For this review, take the finished solid that the model builds, in its own axes (mm). Face numbers are marked on the shaded views. Give positions to 0.01 mm unless a question says otherwise; leave off trailing zeros. Order: outer loops, then holes, each group sorted by start corner. A loop starts at its lowest first (then second) coordinate and runs counter-clockwise, first axis right, second up.
Autodesk Inventor part; units mm, degrees
ref_plane "Work Plane1" through (15.24, 0, -4.7625) normal (0, 0, 1) x (1, 0, 0)
ref_plane "YZ Plane" through (0, 0, 0) normal (1, 0, 0) x (0, 1, 0)
ref_plane "XZ Plane" through (0, 0, 0) normal (0, 1, 0) x (-1, 0, 0)
sketch "Sketch1" plane through (0, 0, 0) normal (0, 1, 0) x (-1, 0, 0)
  line L0 (0, 0) -> (0, -9.525)
  line L1 (-15.24, 4.2545) -> (-15.24, -13.7795)
  line L2 (0, 0) -> (-15.24, 4.2545)
  line L3 (0, -9.525) -> (-15.24, -13.7795)
  line L4 (-15.24, 4.2545) -> (-19.05, 4.2545)
  line L5 (-19.05, 4.2545) -> (-19.05, 2.9845)
  line L6 (-19.05, 2.9845) -> (-15.24, 2.9845)
  line L7 (-15.24, 2.9845) -> (-15.24, 4.2545)
  line L8 (-15.24, -13.7795) -> (-19.05, -13.7795)
  line L9 (-19.05, -13.7795) -> (-19.05, -12.5095)
  line L10 (-19.05, -12.5095) -> (-15.24, -12.5095)
  line L11 (-15.24, -12.5095) -> (-15.24, -13.7795)
  line L12 (0, 0) -> (0, 3.175)
  line L13 (-15.24, 4.2545) -> (-15.24, 7.4295)
  line L14 (0, -9.525) -> (0, -12.7)
  line L15 (-15.24, -13.7795) -> (-15.24, -16.9545)
  line L16 (-15.24, -16.9545) -> (0, -12.7)
  line L17 (0, 3.175) -> (-15.24, 7.4295)
  line L18 (-15.24, 7.4295) -> (-34.29, 7.4295)
  line L19 (-19.05, 4.2545) -> (-34.29, 4.2545)
  line L20 (-34.29, 4.2545) -> (-34.29, 7.4295)
  line L21 (-15.24, -16.9545) -> (-34.29, -16.9545)
  line L22 (-34.29, -16.9545) -> (-34.29, -13.7795)
  line L23 (-34.29, -13.7795) -> (-19.05, -13.7795)
  line L24 (-34.29, 7.4295) -> (-37.465, 7.4295)
  line L25 (-37.465, 7.4295) -> (-37.465, -17.5895)
  line L26 (-37.465, -17.5895) -> (-34.29, -17.5895)
  line L27 (-34.29, -17.5895) -> (-34.29, 7.4295)
  line L28 (-15.24, -13.7795) -> (-34.29, -13.7795)
  line L29 (-34.29, -13.7795) -> (-34.29, 4.2545)
  line L30 (-34.29, 4.2545) -> (-15.24, 4.2545)
  line L31 (-15.24, 4.2545) -> (-15.24, -13.7795)
  line L32 (-15.24, 4.2545) -> (-34.29, 4.2545)
  line L33 (-34.29, 4.2545) -> (-34.29, 7.4295)
  line L34 (-34.29, 7.4295) -> (-15.24, 7.4295)
  line L35 (-15.24, 7.4295) -> (-15.24, 4.2545)
  line L36 (-15.24, -7.5565) -> (-22.86, -7.5565)
  line L37 (-22.86, -7.5565) -> (-22.86, -1.9685)
  line L38 (-22.86, -1.9685) -> (-15.24, -1.9685)
  line L39 (-15.24, -1.9685) -> (-15.24, -7.5565)
  dimension "d0" = 9.525
  dimension "d1" = 15.24
  dimension "d2" = 18.034
  dimension "d3" = 4.2545
  dimension "d4" = 3.81
  dimension "d5" = 1.27
  dimension "d6" = 3.81
  dimension "d7" = 1.27
  dimension "d8" = 3.175
  dimension "d9" = 3.175
  dimension "d10" = 3.175
  dimension "d11" = 3.175
  dimension "d12" = 19.05
  dimension "d13" = 3.175
  dimension "d30" = 7.62
  dimension "d31" = 5.588
  dimension "d32" = 6.223
extrude "Extrusion6" add sketch "Sketch1" along normal blind 5.588 contours L0 L3 L1 L2 | L1 L36 L37 L38
sketch "Sketch5" plane through (0, 5.588, 0) normal (0, 1, 0) x (1, 0, 0)
  circle A0 centre (8.636, 4.7625) radius 1.5875
  line L0 (0, 9.525) -> (0, 0)
  dimension "d35" = 3.175
  dimension "d36" = 8.636
extrude "Extrusion7" cut sketch "Sketch5" against normal blind 5.588
sketch "Sketch6" plane through (15.24, 0, 4.2545) normal (1, 0, 0) x (0, 0, -1)
  line L0 (6.223, 0) -> (6.223, 5.588)
  line L1 (0, 5.588) -> (6.223, 5.588)
  line L2 (0, 0) -> (0, 5.588)
  line L3 (0, 0) -> (6.223, 0)
  line L4 (11.811, 5.588) -> (11.811, 0)
  line L5 (11.811, 0) -> (18.034, 0)
  line L6 (18.034, 0) -> (18.034, 5.588)
  line L7 (11.811, 5.588) -> (18.034, 5.588)
  circle A0 centre (1.863, 2.794) radius 0.381
  circle A1 centre (4.4524, 2.794) radius 0.381
  line L8 (6.223, 5.588) -> (11.811, 5.588)
  line L9 (9.017, 5.588) -> (9.017, 8.4963)
  circle A2 centre (16.171, 2.794) radius 0.381
  circle A3 centre (13.5816, 2.794) radius 0.381
  point P0 (4.2545, 0)
  dimension "d39" = 0.762
  dimension "d40" = 0.762
extrude "Extrusion8" add sketch "Sketch6" along normal blind 12.7 contours A0 | A1 | A2 | A3
ref_plane "Work Plane1" through (15.24, 0, -4.7625) normal (0, 0, 1) x (1, 0, 0)
equation "\"d3\" = -0.5 * d0 + 0.5 * d2"
equation "\"d32\" = -0.5 * d31 + 0.5 * d2"
properties part number "photoTransistor" material "ABS Plastic"
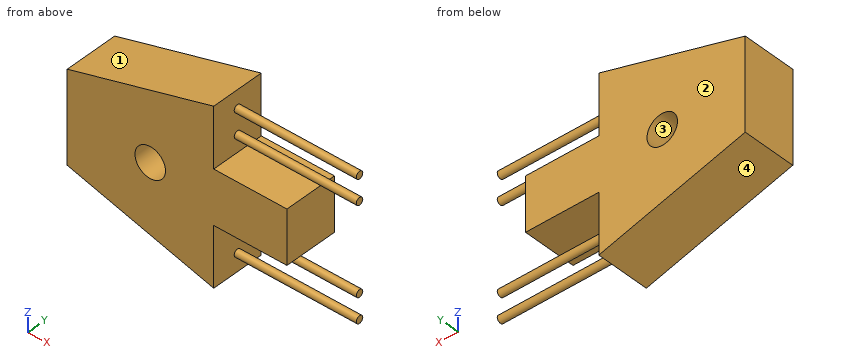
1) Clearance check with flat-ended pins moving along their axes: pin 1 (1 mm diameter, centred on y = 2, z = -10, fed in from +X); pin 2 (3 mm diameter, centred on x = 18.5, y = 2.5, fed in from +Z). State where each tip first meets the part, or that it passes through.
Answer sheet:
pin 1: stops at x = 15.24
pin 2: stops at z = 2.77
2) To check wall thickness, follow line 1 (X direction, y = 3.6, z = -9.25); line 2 (X direction, y = 3.6, z = -2.75); line 3 (Z direction, x = 22.25, y = 4.7). State the ranges of each line that lie inside material, in increasing order.
Answer sheet:
line 1: x = 0 to 15.24
line 2: x = 0 to 22.86
line 3: z = -7.56 to -1.97
3) We need section D-D on x = 18. Give the boundary of the cut face in (y, z), then the cut area to 3 significant figures.
Answer sheet:
outline: (0, -7.56) - (5.59, -7.56) - (5.59, -1.97) - (0, -1.97) - close; circle Ø0.76 at (2.79, -11.92); circle Ø0.76 at (2.79, -9.33); circle Ø0.76 at (2.79, -0.2); circle Ø0.76 at (2.79, 2.39)
area: 33.0 mm2
4) Draft analysis for pull direction Z (two halves, no side actions). For the marked faces 1, 2, 3 and 4, state which applies: +Z half, -Z half, draft (parallel to the pull), parting line (faces both ways), or undercut.
Answer sheet:
face 1: +Z half
face 2: draft
face 3: undercut
face 4: -Z half
5) We need section B-B on z = -4.25. Give the boundary of the cut face in (x, y).
Answer sheet:
outline: (0, 0) - (7.13, 0) - (7.13, 5.59) - (0, 5.59) - close; (10.14, 0) - (22.86, 0) - (22.86, 5.59) - (10.14, 5.59) - close
6) We need section A-A on x = 8. Give the boundary of the cut face in (y, z).
Answer sheet:
outline: (0, -11.76) - (5.59, -11.76) - (5.59, -6.22) - (0, -6.22) - close; (0, -3.31) - (5.59, -3.31) - (5.59, 2.23) - (0, 2.23) - close
7) We need section C-C on y = 0.55. Give the boundary of the cut face in (x, z) (1 decimal).
Answer sheet:
outline: (0, -9.5) - (15.2, -13.8) - (15.2, -7.6) - (22.9, -7.6) - (22.9, -2) - (15.2, -2) - (15.2, 4.3) - (0, 0) - close; hole circle Ø3.2 at (8.6, -4.8)
